Check sheet for the modelled part. Datum: model origin and axes. Units: mm. Face numbers are marked on the shaded views. A direction names the side the tool comes from. Give positions to 0.01 mm unless a question says otherwise; leave off trailing zeros. Order: outer loops, then holes, each group sorted by start corner. A loop starts at its lowest first (then second) coordinate and runs counter-clockwise, first axis right, second up.
Item 1: Material ranges on line 1 along Y through (x, z) = (5.75, 0) (3 decimals); line 2 along Y through (x, z) = (-2, 0); line 3 along Z through (x, y) = (4, 0), recorded low to high.
Item 2: Sectioned sample at A-A on z = 0. Record the boundary of the cut face in (x, y) (1 decimal).
Item 3: Gauge pin test, flat ends, axial feed: P1, Ø10, axis at y = 1.5, z = 6.5, coming from the +X side; P2, Ø2, axis at x = 6, z = -8, coming from the -Y side (3 decimals); P3, Ø10, axis at x = -6, y = -3, coming from the +Z side. Record the tip position at first contact, or that the pin passes through.
Item 4: Sectioned sample at D-D on y = -5.75. Record the boundary of the cut face in (x, z) (1 decimal), and give its area (3 significant figures).
Item 5: Sectioned sample at C-C on y = 0. Record the boundary of the cut face in (x, z) (1 decimal).
Item 6: Release check for a two-part mould opening along Z. For the marked faces 1, 2 and 3 record: released by +Z, released by -Z, zero draft, split by the parting line, or undercut.
Item 7: Sectioned sample at B-B on x = 0. Record the boundary of the cut face in (y, z) (1 decimal), and give its area (3 significant figures).
Item 8: Access from +Z, -Z, +X, -X, +Y, -Y to the whole of each face (thin tool, end or side, straight path). Record for the marked faces 4, 5 and 6.
from build123d import *

# Parameters (mm, degrees)
F0_R     = 11.1125
F0_R_2   = 2.921
F1_DEPTH = 9.525
F2_DEPTH = 12.7
F3_R     = 2.921
F4_DEPTH = 27.813


with BuildPart() as f1:
    # F0 (on Front) → F1 (new body, symmetric)
    with BuildSketch(Plane.XZ):
        Circle(F0_R)
        Circle(F0_R_2, mode=Mode.SUBTRACT)
    extrude(amount=F1_DEPTH, both=True)

    # F0 (on Front) → F2 (join, symmetric)
    with BuildSketch(Plane.XZ):
        Circle(F0_R_2)
    extrude(amount=F2_DEPTH, both=True)

    # F3 (on Right) → F4 (cut, symmetric)
    with BuildSketch(Plane.YZ):
        Circle(F3_R)
    extrude(amount=F4_DEPTH, both=True, mode=Mode.SUBTRACT)


solid = f1.part
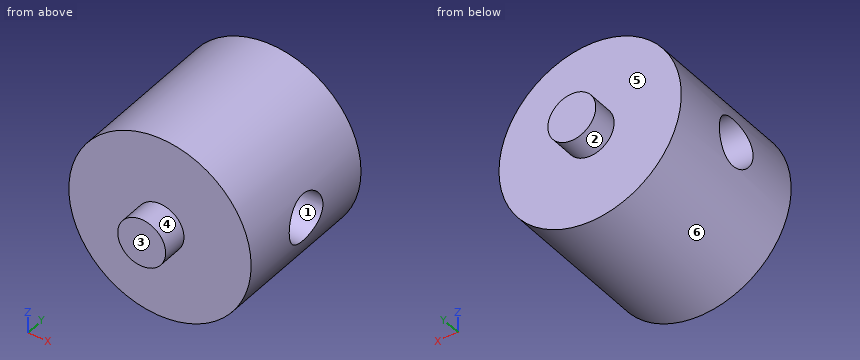
Report:
1. line 1: y = -9.525 to -2.921, 2.921 to 9.525
1. line 2: y = -12.7 to -2.92, 2.92 to 12.7
1. line 3: z = -10.37 to -2.92, 2.92 to 10.37
2. outline: (-11.1, -9.5) - (-2.9, -9.5) - (-2.9, -12.7) - (2.9, -12.7) - (2.9, -9.5) - (11.1, -9.5) - (11.1, -2.9) - (-11.1, -2.9) - close; (-11.1, 2.9) - (11.1, 2.9) - (11.1, 9.5) - (2.9, 9.5) - (2.9, 12.7) - (-2.9, 12.7) - (-2.9, 9.5) - (-11.1, 9.5) - close
3. P1: stops at x = 11
3. P2: stops at y = -9.525
3. P3: stops at z = 11.07
4. outline: circle Ø22.2 at (0, 0)
4. area: 388 mm2
5. outline: (-10.7, -2.9) arc R11.1 ccw to (10.7, -2.9) - close; (-10.7, 2.9) - (10.7, 2.9) arc R11.1 ccw to start
6. face 1: undercut
6. face 2: split by the parting line
6. face 3: zero draft
7. outline: (-12.7, -2.9) - (-9.5, -2.9) - (-9.5, -11.1) - (9.5, -11.1) - (9.5, -2.9) - (12.7, -2.9) - (12.7, 2.9) - (9.5, 2.9) - (9.5, 11.1) - (-9.5, 11.1) - (-9.5, 2.9) - (-12.7, 2.9) - close; hole circle Ø5.8 at (0, 0)
7. area: 434 mm2
8. face 4: -Y
8. face 5: +Y
8. face 6: +Y, -Y
